The model under review builds one solid part; all positions refer to its coordinate system, in mm. Face numbers are marked on the shaded views. A direction names the side the tool comes from. Give positions to 0.01 mm unless a question says otherwise; leave off trailing zeros. Write each loop counter-clockwise with the first axis right and the second up, starting at its lowest first coordinate (ties: lowest second). Pieces come first, ordered by that corner, then holes.
from build123d import *

# Parameters (mm, degrees)
RADYUS1_R               = 0.5
KES_EKSTR_ZYON1_START   = -4
KES_EKSTR_ZYON1_DEPTH   = 4
DAIRESEL_KAPLAMA1_COUNT = 11


with BuildPart() as part:
    # Çizim1 → Döndür1 (revolve)
    with BuildSketch(Plane.XY, mode=Mode.PRIVATE) as d_nd_r1_sk:
        Polygon((0, 0), (0, 26.1), (1, 26.1), (1, 25.939294597), (2, 25.939294597), (2, 21.939294597), (1, 21.939294597), (1, 20), (4, 20), (4, 0), align=None)
    revolve(d_nd_r1_sk.sketch.rotate(Axis((0, 0, 0), (0, 1, 0)), 90), axis=Axis((0, 0, 0), (0, 1, 0)))

    # Radyus1
    radyus1_edges = [part.edges().sort_by_distance(p)[0] for p in [
        (0, 0, 4),
        (0, 20, 4),
    ]]
    fillet(radyus1_edges, radius=RADYUS1_R)

    # Çizim2 → Kes-Ekstrüzyon1 (cut)
    with BuildSketch(Plane(origin=(0, 25.939294597, 0), x_dir=(1, 0, 0), z_dir=(0, 1, 0)).offset(KES_EKSTR_ZYON1_START)):
        with BuildLine():
            ThreePointArc((0.5, 1.936491673), (0, 2), (-0.5, 1.936491673))
            ThreePointArc((-0.5, 1.936491673), (-0.266031544, 1.636956648), (-0.092954447, 1.298568131))
            ThreePointArc((-0.092954447, 1.298568131), (0, 1.235439134), (0.092954447, 1.298568131))
            ThreePointArc((0.092954447, 1.298568131), (0.266031544, 1.636956648), (0.5, 1.936491673))
        make_face()
    kes_ekstr_zyon1 = extrude(amount=KES_EKSTR_ZYON1_DEPTH, mode=Mode.SUBTRACT)

    # Dairesel Kaplama1: Kes-Ekstrüzyon1 ×11 about axis
    dairesel_kaplama1_axis = Axis((0, 0, 0), (0, 1, 0))
    for i in range(1, DAIRESEL_KAPLAMA1_COUNT):
        add(kes_ekstr_zyon1.rotate(dairesel_kaplama1_axis, i * 360 / DAIRESEL_KAPLAMA1_COUNT), mode=Mode.SUBTRACT)


solid = part.part
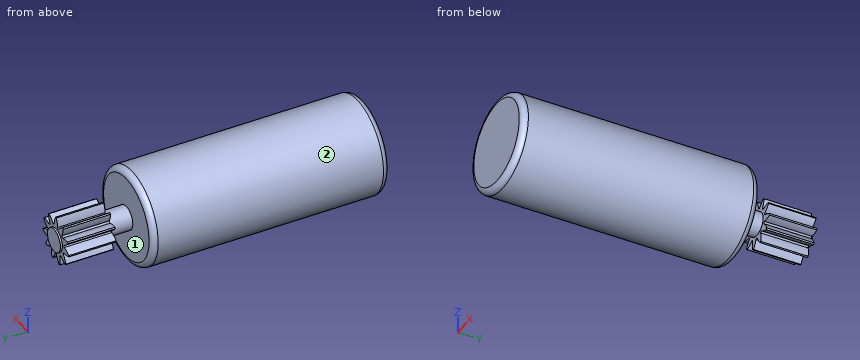
1) Tool access review of the marked faces 1 and 2: name each direction out of +Z, -Z, +X, -X, +Y, -Y from which nothing blocks a thin tool from reaching the whole face with its end or side.
2) To check wall thickness, follow probe 1 along Z at (x, y) = (-1.5, 23.5); probe 2 along Y at (x, z) = (-0.75, 3.5); probe 3 along X at (y, z) = (9.75, 1.25). State the ranges of each line that lie inside material, in increasing order.
3) Consider section A-A, the plane y = 16. Give the boundary of the cut face in (x, z).
Answer block:
1. face 1: none
1. face 2: +Y, -Y
2. probe 1: z = -1.32 to -1.14, -0.45 to 0.03, 0.43 to 0.88
2. probe 2: y = 0.01 to 19.99
2. probe 3: x = -3.8 to 3.8
3. outline: circle Ø8 at (0, 0)
